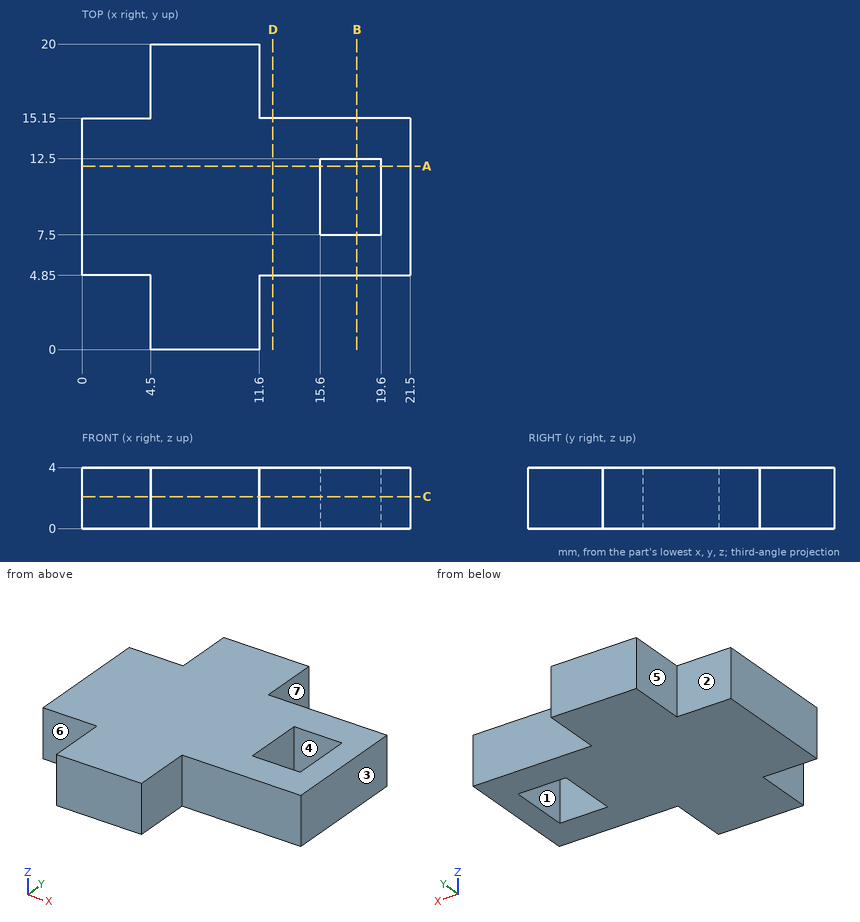
Geometry: see drawing. Coordinates: mm, zero at the bounding-box minimum. A direction names the side the tool comes from. Round coordinates to 2 decimals unless told otherwise and drop trailing zeros. Loops run counter-clockwise (first coordinate to the right, second up) from the corner with the lowest first, then second, coordinate; pieces in that order, holes last. Notation, with made-up numbers: (55, -39) -> (61, -39) arc R12 cw to (61, -18) -> close; hole circle Ø11 at (8.5, 84.5). An arc over 180 degrees is marked (long way). Use one line per item in the form item = value. Start each with the question number.
Item 1: Section query D-D on x = 12.5. Return the cut outline in (y, z).
Item 2: Contact query for flat-ended pins moving along their axis: pin 1 Ø2 at (x, z) = (18, 2) entering from -Y; pin 2 Ø1.2 at (y, z) = (2.5, 2) entering from -X; pin 3 Ø8 at (x, y) = (7.5, 8.5) entering from -Z; pin 4 Ø2 at (y, z) = (18.5, 2.5) entering from +X. Output: stop coordinate, or through.
Item 3: Section query B-B on x = 18. Return the cut outline in (y, z), then the cut area to 3 significant figures.
Item 4: Section query C-C on z = 2.1. Return the cut outline in (x, y), then the cut area to 3 significant figures.
Item 5: Material intervals for L1, parallel to Y at x = 15.75, z = 1.95; L2, parallel to X at y = 10, z = 2.65; L3, parallel to X at y = 4, z = 2.55, sorted ascending. Write a range as from..to.
Item 6: Section query A-A on y = 12. Return the cut outline in (x, z).
Item 7: Set-up query: the marked faces 4, 5, 6 and 7. Return all of +Z, -Z, +X, -X, +Y, -Y with unobstructed straight access to the full face (end or side cutting, diameter ignored); none if empty.
Item 8: Mould query, pull axis Y, two halves, no side actions, for the marked faces 1, 2 and 3. Classes: pulls with the +Y half, pulls with the -Y half, needs draft (parallel to the pull), parting line crosses it, or undercut.
Ans:
q1.outline = (4.85, 0) -> (15.15, 0) -> (15.15, 4) -> (4.85, 4) -> close
q2.pin_1 = 4.85
q2.pin_2 = 4.5
q2.pin_3 = 0
q2.pin_4 = 11.6
q3.outline = (4.85, 0) -> (7.5, 0) -> (7.5, 4) -> (4.85, 4) -> close; (12.5, 0) -> (15.15, 0) -> (15.15, 4) -> (12.5, 4) -> close
q3.area = 21.2 mm^2
q4.outline = (0, 4.85) -> (4.5, 4.85) -> (4.5, 0) -> (11.6, 0) -> (11.6, 4.85) -> (21.5, 4.85) -> (21.5, 15.15) -> (11.6, 15.15) -> (11.6, 20) -> (4.5, 20) -> (4.5, 15.15) -> (0, 15.15) -> close; hole (15.6, 7.5) -> (19.6, 7.5) -> (19.6, 12.5) -> (15.6, 12.5) -> close
q4.area = 270 mm^2
q5.L1 = 4.85..7.5, 12.5..15.15
q5.L2 = 0..15.6, 19.6..21.5
q5.L3 = 4.5..11.6
q6.outline = (0, 0) -> (15.6, 0) -> (15.6, 4) -> (0, 4) -> close; (19.6, 0) -> (21.5, 0) -> (21.5, 4) -> (19.6, 4) -> close
q7.face_4 = +Z, -Z
q7.face_5 = +Z, -Z, -X, +Y
q7.face_6 = +Z, -Z, -X, -Y
q7.face_7 = +Z, -Z, +X, +Y
q8.face_1 = undercut
q8.face_2 = pulls with the +Y half
q8.face_3 = needs draft
